Here's how the part is built. I have some questions about the finished solid (model axes, mm). Face numbers are marked on the shaded views. Round coordinates to 2 decimals unless told otherwise and drop trailing zeros. Write each loop counter-clockwise with the first axis right and the second up, starting at its lowest first coordinate (ties: lowest second). Pieces come first, ordered by that corner, then holes. Notation, with made-up numbers: (20.5, 19.5) - (37.5, 19.5) arc R14 ccw to (37.5, 45.5) - close; hole circle Ø11 at (-16, 6). An arc over 180 degrees is marked (long way). Return JSON: item names as keys, results as strings. Group by question number.
```python
from build123d import *

# Parameters (mm, degrees)
SKETCH1_R           = 4.1
SKETCH1_R_2         = 2
BOSS_EXTRUDE1_DEPTH = 3
FILLET1_R           = 2


with BuildPart() as part:
    # Sketch1 → Boss-Extrude1 (new body)
    with BuildSketch(Plane(origin=(0, 0, 0), x_dir=(1, 0, 0), z_dir=(0, 1, 0))):
        with BuildLine():
            Line((-14, 5.656854249), (-3.333333333, 9.428090416))
            ThreePointArc((-3.333333333, 9.428090416), (0, 10), (3.333333333, 9.428090416))
            Line((3.333333333, 9.428090416), (14, 5.656854249))
            ThreePointArc((14, 5.656854249), (18, 0), (14, -5.656854249))
            Line((14, -5.656854249), (3.333333333, -9.428090416))
            ThreePointArc((3.333333333, -9.428090416), (0, -10), (-3.333333333, -9.428090416))
            Line((-3.333333333, -9.428090416), (-14, -5.656854249))
            ThreePointArc((-14, -5.656854249), (-18, 0), (-14, 5.656854249))
        make_face()
        with Locations(Location((0, 0, 0), (0, 0, 270))):
            Circle(SKETCH1_R, mode=Mode.SUBTRACT)
        with Locations(Location((-12, 0, 0), (0, 0, 270))):
            Circle(SKETCH1_R_2, mode=Mode.SUBTRACT)
        with Locations(Location((12, 0, 0), (0, 0, 270))):
            Circle(SKETCH1_R_2, mode=Mode.SUBTRACT)
    extrude(amount=BOSS_EXTRUDE1_DEPTH)

    # Fillet1
    fillet1_edges = [part.edges().sort_by_distance(p)[0] for p in [
        (0, 3, 10),
        (8.666666667, 3, 7.542472333),
        (18, 3, 0),
        (8.666666667, 3, -7.542472333),
        (0, 3, -10),
        (-8.666666667, 3, -7.542472333),
        (-18, 3, 0),
        (-8.666666667, 3, 7.542472333),
    ]]
    fillet(fillet1_edges, radius=FILLET1_R)


solid = part.part
```
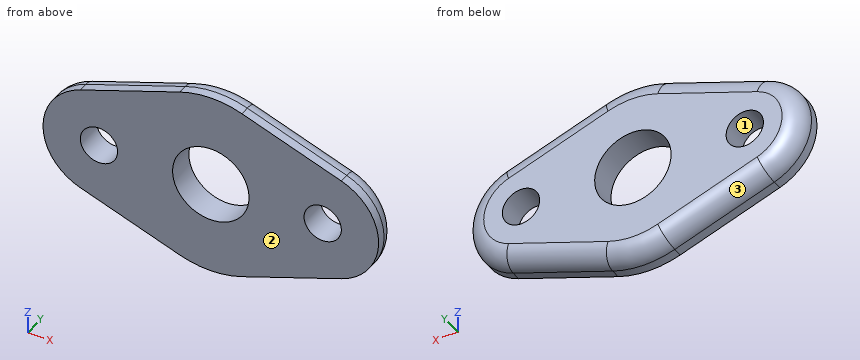
1) Imagine slicing it at D-D (y = 2.2). Please give me the cut outline in (x, z).
2) Imagine slicing it at B-B (z = 0). Please give me the cut outline in (x, y), plus the area to 3 significant figures.
3) I need wall thicknesses on line 1 along X through (y, z) = (0.8, 0); line 2 along X through (y, z) = (2.3, 0); line 3 along Z through (x, y) = (-12.5, 0.7). Which ranges of each line are inside material? Lowest first, please.
4) Imagine slicing it at A-A (y = 0.65). Please give me the cut outline in (x, z), plus the area to 3 significant figures.
5) Imagine slicing it at C-C (x = 0). Please give me the cut outline in (y, z).
6) If we mould it in two halves opening along X, with no side actions, what happens to the marked faces 1, 2 and 3? For each: released by +X, released by -X, zero draft, split by the parting line, or undercut.
7) Will this pin go through, and if not, where does the flat tip stop? pin 1 Ø3.5 at (x, z) = (-12, 0) entering from +Y.
Results found:
{
 "1": {"outline": "(-13.87, -5.28) - (-3.2, -9.05) arc R9.6 ccw to (3.2, -9.05) - (13.87, -5.28) arc R5.6 ccw to (13.87, 5.28) - (3.2, 9.05) arc R9.6 ccw to (-3.2, 9.05) - (-13.87, 5.28) arc R5.6 ccw to start; hole circle Ø4 at (-12, 0); hole circle Ø8.2 at (0, 0); hole circle Ø4 at (12, 0)"},
 "2": {"outline": "(-18, 0) - (-14, 0) - (-14, 3) - (-16, 3) arc R2 ccw to (-18, 1) - close; (-10, 0) - (-4.1, 0) - (-4.1, 3) - (-10, 3) - close; (4.1, 0) - (10, 0) - (10, 3) - (4.1, 3) - close; (14, 0) - (18, 0) - (18, 1) arc R2 ccw to (16, 3) - (14, 3) - close", "area": "57.7 mm²"},
 "3": {"line 1": "x = -18 to -14, -10 to -4.1, 4.1 to 10, 14 to 18", "line 2": "x = -17.52 to -14, -10 to -4.1, 4.1 to 10, 14 to 17.52", "line 3": "z = -6.19 to -1.94, 1.94 to 6.19"},
 "4": {"outline": "(-14, -5.66) - (-3.33, -9.43) arc R10 ccw to (3.33, -9.43) - (14, -5.66) arc R6 ccw to (14, 5.66) - (3.33, 9.43) arc R10 ccw to (-3.33, 9.43) - (-14, 5.66) arc R6 ccw to start; hole circle Ø4 at (-12, 0); hole circle Ø8.2 at (0, 0); hole circle Ø4 at (12, 0)", "area": "441 mm²"},
 "5": {"outline": "(0, -10) - (1, -10) arc R2 ccw to (3, -8) - (3, -4.1) - (0, -4.1) - close; (0, 4.1) - (3, 4.1) - (3, 8) arc R2 ccw to (1, 10) - (0, 10) - close"},
 "6": {"face 1": "undercut", "face 2": "zero draft", "face 3": "released by -X"},
 "7": {"pin 1": "passes through"}
}
